from build123d import *

# Parameters (mm, degrees)
BOSS_EXTRUDE1_DEPTH = 12
CHAMFER1_SIZE       = 12
SKETCH2_R           = 4
SKETCH2_R_2         = 10
CUT_EXTRUDE1_DEPTH  = 609.394608786


with BuildPart() as part:
    # Sketch1 → Boss-Extrude1 (new body)
    with BuildSketch(Plane.XY):
        with BuildLine():
            Line((0, 0), (0, -10))
            Line((0, -10), (40, -10))
            ThreePointArc((40, -10), (48.819660113, -2.639320225), (60, 0))
            Line((60, 0), (165, 0))
            ThreePointArc((165, 0), (176.180339887, -2.639320225), (185, -10))
            Line((185, -10), (415, -10))
            ThreePointArc((415, -10), (423.819660113, -2.639320225), (435, 0))
            Line((435, 0), (540, 0))
            ThreePointArc((540, 0), (551.180339887, -2.639320225), (560, -10))
            Line((560, -10), (600, -10))
            Line((600, -10), (600, 0))
            Line((600, 0), (600, 100))
            Line((600, 100), (0, 100))
            Line((0, 100), (0, 0))
        make_face()
    extrude(amount=BOSS_EXTRUDE1_DEPTH)

    # Chamfer1
    chamfer1_edges = [part.edges().sort_by_distance(p)[0] for p in [
        (300, 100, 12),
        (600, 45, 12),
        (0, 45, 12),
    ]]
    chamfer(chamfer1_edges, length=CHAMFER1_SIZE - 0.0001)  # a hair under: the kernel refuses the full size

    # Sketch2 → Cut-Extrude1 (cut, through all)
    with BuildSketch(Plane(origin=(0, 0, 0), x_dir=(-1, 0, 0), z_dir=(0, 0, -1))):
        with Locations((-335, 55)):
            Circle(SKETCH2_R)
        with Locations((-300, 35)):
            Circle(SKETCH2_R_2)
        with Locations((-265, 55)):
            Circle(SKETCH2_R)
        with Locations((-335, 10)):
            Circle(SKETCH2_R)
        with Locations((-265, 10)):
            Circle(SKETCH2_R)
    extrude(amount=-CUT_EXTRUDE1_DEPTH, mode=Mode.SUBTRACT)


solid = part.part
Could you check a few things on this model? Use its own coordinates, in mm. A direction names the side the tool comes from. Round coordinates to 2 decimals unless told otherwise and drop trailing zeros. Write each loop counter-clockwise with the first axis right and the second up, starting at its lowest first coordinate (ties: lowest second). Pieces come first, ordered by that corner, then holes. Notation, with made-up numbers: (44.25, 68) -> (68.25, 68) arc R5 ccw to (68.25, 75) -> close; hole circle Ø9 at (15, -35). An arc over 180 degrees is marked (long way). Use a Markdown table: item, result.
1. Which directions (+Z, -Z, +X, -X, +Y, -Y) give clear straight access to the entire face, cutting with the end or side of a thin tool? Please do faces 5 (the face through (575, -10, 6)), 6 (the face through (423.7, -2.7, 5.9)).
Answer key:
| item | result |
|---|---|
| face 5 | +Z, -Z, +X, -X, -Y |
| face 6 | +Z, -Z, -Y |
2. We'd pull the mould along X, two halves only. Please class faces 1 (the face through (487, 0, 6)), 2 (the face through (6, 46, 6)), 3 (the face through (594, 44, 6)), 4 (the face through (298, -10, 6)): +X half, -X half, draft (parallel to the pull), parting line (faces both ways), or undercut.
Answer key:
| item | result |
|---|---|
| face 1 | undercut |
| face 2 | -X half |
| face 3 | +X half |
| face 4 | draft |
3. For pin 1 Ø13 at (x, y) = (265, 10) entering from -Z; pin 2 Ø7 at (x, y) = (265, 55) entering from -Z; pin 3 Ø3.5 at (x, z) = (101.5, 4.5) entering from -Y; pin 4 Ø5 at (x, z) = (372, 6.5) entering from +Y, each with a flat end and sliding along its axis, tell me the tip position at first contact or that it passes through.
Answer key:
| item | result |
|---|---|
| pin 1 | stops at z = 0 |
| pin 2 | passes through |
| pin 3 | stops at y = 0 |
| pin 4 | stops at y = 96 |
4. Please list where these lines run through material, in increasing order: probe 1 along Y at (x, z) = (265, 3.75); probe 2 along Y at (x, z) = (265, 7); probe 3 along X at (y, z) = (7.5, 2.5).
Answer key:
| item | result |
|---|---|
| probe 1 | y = -10 to 6, 14 to 51, 59 to 96.25 |
| probe 2 | y = -10 to 6, 14 to 51, 59 to 93 |
| probe 3 | x = 2.5 to 261.88, 268.12 to 331.88, 338.12 to 597.5 |
5. If we section it at C-C (z = 6.75): List the corners of the cut face in (x, y) for me.
Answer key:
| item | result |
|---|---|
| outline | (6.75, -10) -> (40, -10) arc R25 cw to (60, 0) -> (165, 0) arc R25 cw to (185, -10) -> (415, -10) arc R25 cw to (435, 0) -> (540, 0) arc R25 cw to (560, -10) -> (593.25, -10) -> (593.25, 93.25) -> (6.75, 93.25) -> close; hole circle Ø8 at (265, 10); hole circle Ø8 at (265, 55); hole circle Ø20 at (300, 35); hole circle Ø8 at (335, 10); hole circle Ø8 at (335, 55) |
